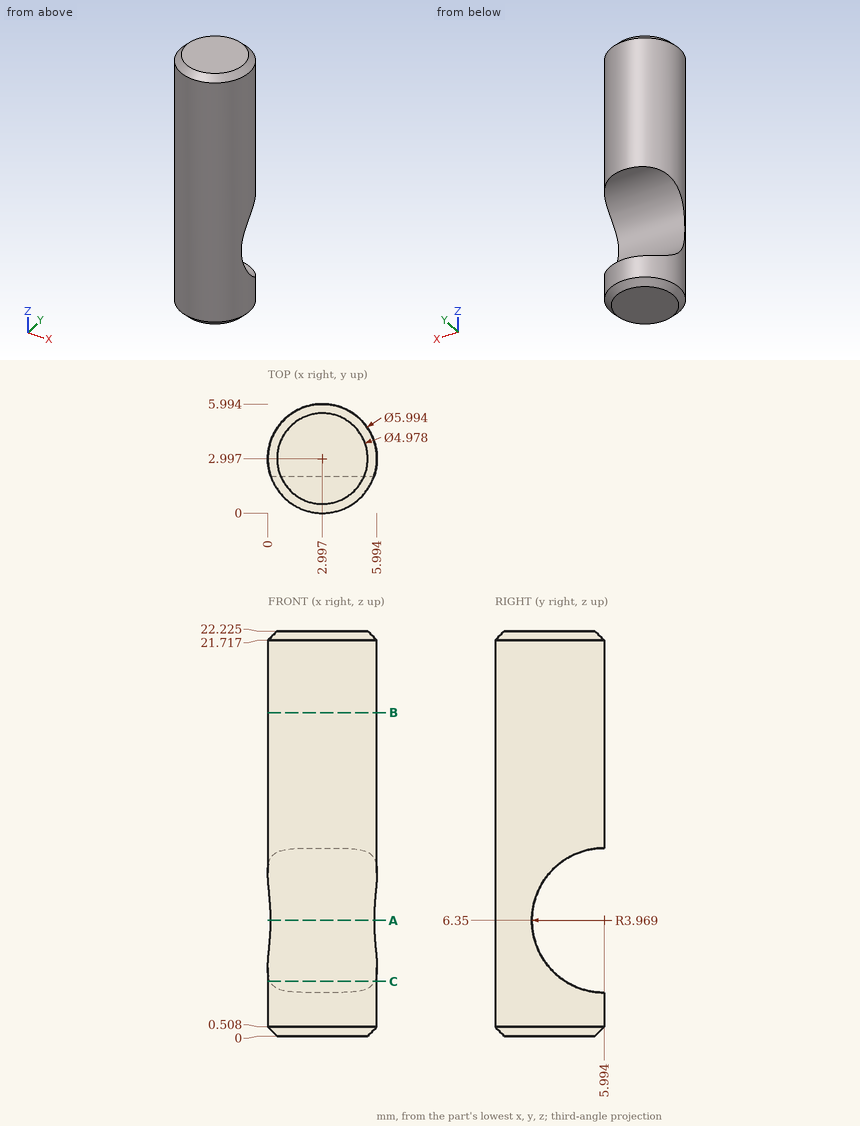
Here's the drawing with two shaded views (mm, measured from the low corner). I have some questions. Give positions to 0.01 mm unless a question says otherwise; leave off trailing zeros. Order: outer loops, then holes, each group sorted by start corner. A loop starts at its lowest first (then second) coordinate and runs counter-clockwise, first axis right, second up.
Q1. Suppose I cut it at C-C, the plane z = 3. Write out the boundary of the cut face in (x, y) (1 decimal).
Q2. If I drill on line 1 along Z through (x, y) = (2.1, 4.7) (1 decimal); line 2 along X through (y, z) = (3.15, 9.25); line 3 along Z through (x, y) = (2.55, 3.8) (1 decimal), over which ranges is the centre line in solid material (lowest first)?
Q3. Suppose I cut it at A-A, the plane z = 6.35. Write out the boundary of the cut face in (x, y) (1 decimal).
Q4. Suppose I cut it at B-B, the plane z = 17.75. Write out the boundary of the cut face in (x, y) (1 decimal), and give its area (3 significant figures).
Q5. I'm going to push a flat-ended pin straight in: P1, Ø1.5, axis at x = 2, z = 9, coming from the +Y side (1 decimal). Where does the tip first touch, or does it pass through?
Solution:
1. outline: (0.1, 3.9) arc R3 ccw (long way) to (5.9, 3.9) - close
2. line 1: z = 0 to 2.6, 10.1 to 22.2
2. line 2: x = 0 to 5.99
2. line 3: z = 0 to 3, 9.7 to 22.2
3. outline: (0.2, 2) arc R3 ccw to (5.8, 2) - close
4. outline: circle Ø6 at (3, 3)
4. area: 28.2 mm2
5. P1: stops at y = 3.9
